Answer from the drawing. Dimensions are ordinates in mm from the lowest x, y and z of the part. Give positions to 0.01 mm unless a question says otherwise; leave off trailing zeros. Write each loop counter-clockwise with the first axis right and the second up, starting at its lowest first coordinate (ties: lowest second). Pieces come first, ordered by that corner, then holes.
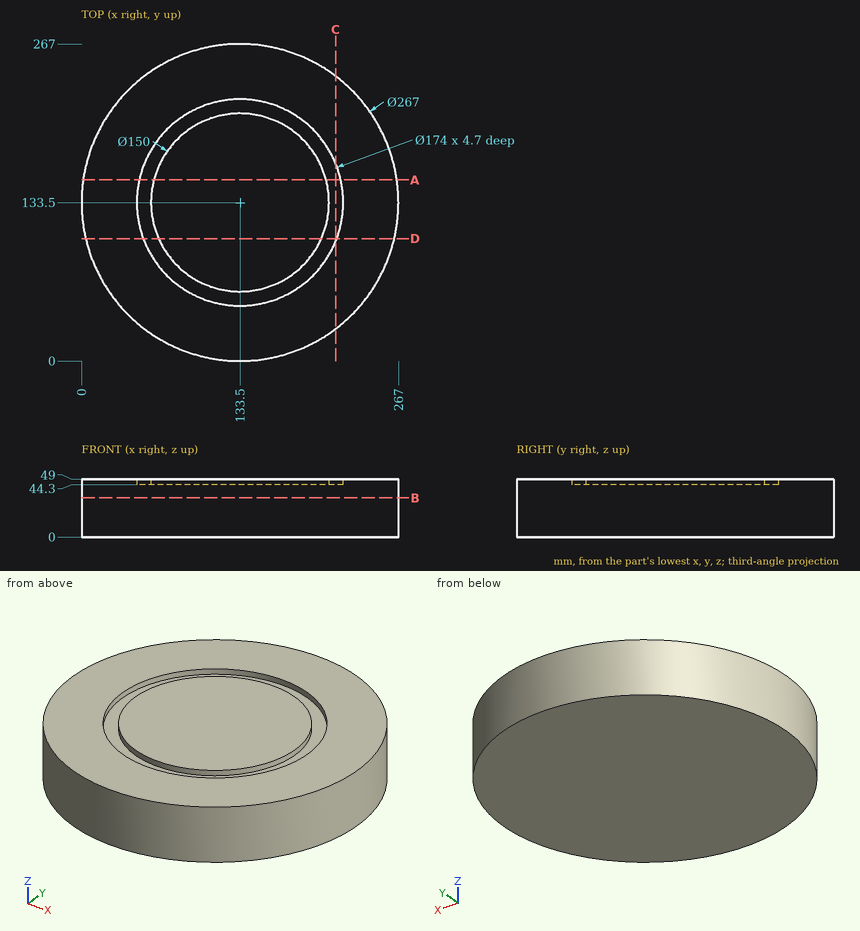
Item 1: A cutting plane is placed at D-D, the plane y = 103. Give the vertices of the cut face in (x, z).
Conclusion:
outline: (3.53, 0) - (263.47, 0) - (263.47, 49) - (214.98, 49) - (214.98, 44.3) - (202.02, 44.3) - (202.02, 49) - (64.98, 49) - (64.98, 44.3) - (52.02, 44.3) - (52.02, 49) - (3.53, 49) - close
Item 2: Consider probe 1 along Y at (x, z) = (133.5, 47.7); probe 2 along Z at (x, y) = (53, 142.5); probe 3 along Y at (x, z) = (164.5, 30.5). Determine where each line is inside the solid, lowest interval first.
Conclusion:
probe 1: y = 0 to 46.5, 58.5 to 208.5, 220.5 to 267
probe 2: z = 0 to 44.3
probe 3: y = 3.65 to 263.35
Item 3: A cutting plane is placed at B-B, the plane z = 33. Give the vertices of the cut face in (x, y), plus the area to 3 significant figures.
Conclusion:
outline: circle Ø267 at (133.5, 133.5)
area: 56,000 mm2
Item 4: A cutting plane is placed at C-C, the plane x = 214. Give the vertices of the cut face in (y, z).
Conclusion:
outline: (27, 0) - (240, 0) - (240, 49) - (166.5, 49) - (166.5, 44.3) - (100.5, 44.3) - (100.5, 49) - (27, 49) - close
Item 5: Each of these flat-tipped pins is pushed along its axis until it touches: P1, Ø1.5, axis at x = 211.5, y = 149.5, coming from the +Z side; P2, Ø1.5, axis at y = 103, z = 18.5, coming from the -X side; P3, Ø4, axis at x = 98, z = 33.5, coming from the -Y side. Where does it stop, or does it pass through?
Conclusion:
P1: stops at z = 44.3
P2: stops at x = 3.36
P3: stops at y = 4.27
Item 6: A cutting plane is placed at A-A, the plane y = 152.5. Give the vertices of the cut face in (x, z), plus the area to 3 significant figures.
Conclusion:
outline: (1.36, 0) - (265.64, 0) - (265.64, 49) - (218.4, 49) - (218.4, 44.3) - (206.05, 44.3) - (206.05, 49) - (60.95, 49) - (60.95, 44.3) - (48.6, 44.3) - (48.6, 49) - (1.36, 49) - close
area: 12,800 mm2
